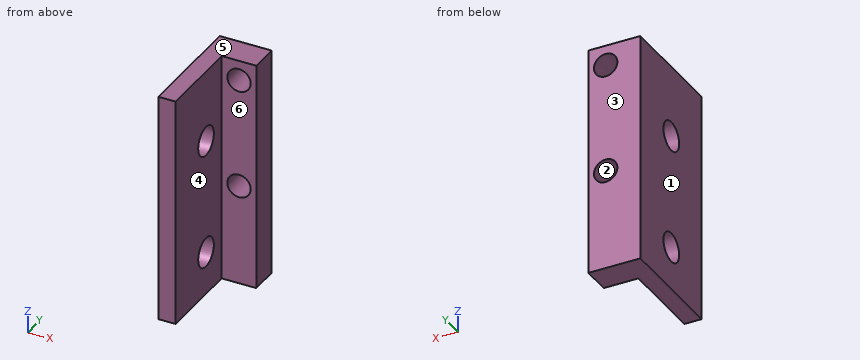
```python
from build123d import *

# Parameters (mm, degrees)
SKETCH1_W           = 9
SKETCH1_H           = 40
SKETCH1_R           = 2.025
BOSS_EXTRUDE1_DEPTH = 5
SKETCH2_W           = 3
SKETCH2_H           = 40
BOSS_EXTRUDE2_DEPTH = 15
SKETCH3_R           = 2.55
CUT_EXTRUDE1_DEPTH  = 46.122056691


with BuildPart() as part:
    # Sketch1 → Boss-Extrude1 (new body)
    with BuildSketch(Plane(origin=(0, 0, 0), x_dir=(1, 0, 0), z_dir=(0, 1, 0))):
        with Locations((4.5, 20)):
            Rectangle(SKETCH1_W, SKETCH1_H)
        with Locations(Location((6, 3.499356869, 0), (0, 0, 270))):
            Circle(SKETCH1_R, mode=Mode.SUBTRACT)
        with Locations(Location((6, 22.499356869, 0), (0, 0, 270))):
            Circle(SKETCH1_R, mode=Mode.SUBTRACT)
    extrude(amount=-BOSS_EXTRUDE1_DEPTH)

    # Sketch2 → Boss-Extrude2 (add)
    with BuildSketch(Plane.XZ.offset(5)):
        with Locations((1.5, -20)):
            Rectangle(SKETCH2_W, SKETCH2_H)
    extrude(amount=BOSS_EXTRUDE2_DEPTH)

    # Sketch3 → Cut-Extrude1 (cut, through all)
    with BuildSketch(Plane(origin=(3, 0, 0), x_dir=(0, 0, -1), z_dir=(1, 0, 0))):
        with Locations((12.5, -10.1)):
            Circle(SKETCH3_R)
        with Locations((32.5, -10.1)):
            Circle(SKETCH3_R)
    extrude(amount=-CUT_EXTRUDE1_DEPTH, mode=Mode.SUBTRACT)


solid = part.part
```
Read the model definition and answer for the solid it produces. Units are mm, in the model's axes. Face numbers are marked on the shaded views. A direction names the side the tool comes from. Round coordinates to 2 decimals unless told otherwise and drop trailing zeros. Write each loop counter-clockwise with the first axis right and the second up, starting at its lowest first coordinate (ties: lowest second). Pieces come first, ordered by that corner, then holes. Notation, with made-up numbers: (64.25, 12) - (115.25, 12) arc R13 ccw to (115.25, 18) - close; hole circle Ø1 at (20.5, 44). An arc over 180 degrees is marked (long way). Use CSV: the item, a comma, the result in double quotes.
Q1. Find section B-B, the plane y = -10.1. Write down the section's boundary in (x, z).
Values:
outline,"(0, -40) - (3, -40) - (3, -35.05) - (0, -35.05) - close; (0, -29.95) - (3, -29.95) - (3, -15.05) - (0, -15.05) - close; (0, -9.95) - (3, -9.95) - (3, 0) - (0, 0) - close"
Q2. A tool of negligible diameter and unlimited length cuts with its end or side. For the marked faces 5 and 6, from which of +Z, -Z, +X, -X, +Y, -Y can it reach the whole face along a straight path? Write none if from no direction.
Values:
face 5,"+Z, +X, -X, +Y, -Y"
face 6,"+Z, -Z, +X, -Y"
Q3. Find section C-C, the plane z = -12.5. Write down the section's boundary in (x, y), then the cut area to 3 significant figures.
Values:
outline,"(0, -20) - (3, -20) - (3, -12.65) - (0, -12.65) - close; (0, -7.55) - (3, -7.55) - (3, -5) - (9, -5) - (9, 0) - (0, 0) - close"
area,"74.7 mm²"
Q4. Straight lines are drawn through the part: line 1 along X through (y, z) = (-6.75, -4); line 2 along Y through (x, z) = (8.25, -31); line 3 along Z through (x, y) = (4.25, -3.25). For each, find the intervals that lie inside material, in ascending order.
Values:
line 1,"x = 0 to 3"
line 2,"y = -5 to 0"
line 3,"z = -40 to -23.52, -21.48 to -4.52, -2.48 to 0"
Q5. Find section D-D, the plane x = 8.5. Write down the section's boundary in (y, z), then the cut area to 3 significant figures.
Values:
outline,"(-5, -40) - (0, -40) - (0, 0) - (-5, 0) - close"
area,"200 mm²"
Q6. Find section A-A, the plane x = 6. Write down the section's boundary in (y, z), then the cut area to 4 significant figures.
Values:
outline,"(-5, -40) - (0, -40) - (0, -24.52) - (-5, -24.52) - close; (-5, -20.47) - (0, -20.47) - (0, -5.52) - (-5, -5.52) - close; (-5, -1.47) - (0, -1.47) - (0, 0) - (-5, 0) - close"
area,"159.5 mm²"
Q7. Each of these flat-tipped pins is pushed along its axis until it touches: pin 1 Ø4.5 at (x, z) = (6, -3.5) entering from +Y; pin 2 Ø2 at (y, z) = (-15, -15) entering from +X; pin 3 Ø3 at (y, z) = (-10.1, -12.5) entering from -X; pin 4 Ø5 at (x, z) = (6.5, -16.5) entering from -Y. Where does it stop, or does it pass through?
Values:
pin 1,"stops at y = 0"
pin 2,"stops at x = 3"
pin 3,"passes through"
pin 4,"stops at y = -5"
Q8. Determine the mould class of the marked faces 1, 2, 3 and 4 for opening direction X: +X half, -X half, draft (parallel to the pull), parting line (faces both ways), or undercut.
Values:
face 1,"-X half"
face 2,"undercut"
face 3,"draft"
face 4,"+X half"
